Can you work these out from the model? Positions are in its coordinate system, mm. A direction names the side the tool comes from. Give positions to 0.01 mm unless a question says otherwise; leave off trailing zeros. Write each loop counter-clockwise with the first axis right and the second up, starting at its lowest first coordinate (ties: lowest second). Pieces come first, ordered by that corner, then holes.
1. Thinking about a two-plate mould opening in Y: for faces 1 (the flat face through (4, 0, 2)), 2 (the cylindrical face through (13.768, 5.555, 2.465)), 3 (the flat face through (4, 14, 0)), which applies, pulls with the +Y half, pulls with the -Y half, needs draft (parallel to the pull), parting line crosses it, or undercut?
2. On a 3-axis mill with a long thin cutter (end or side, diameter ignored), from which of +Z, -Z, +X, -X, +Y, -Y can I reach the whole of each face in a straight line? I mean faces 4 (the flat face through (28.266, 2, 2)), 5 (the flat face through (-22, 5, 2)), 6 (the flat face through (-24.734, 10, 2)), 7 (the flat face through (28.266, 18, 2)), 8 (the cylindrical face through (-15.303, 17.451, 2.465)). Say none if no direction works.
3. Suppose I cut it at C-C (z = 1.5). Please give me the cut outline in (x, y), and give its area (3 significant figures).
4. Suppose I cut it at B-B (x = -17.5). Please give me the cut outline in (y, z).
5. Suppose I cut it at A-A (y = 17). Please give me the cut outline in (x, z), and give its area (3 significant figures).
6. I'm going to push flat-ended pins straight in: pin 1 (1.5 mm diameter, centred on x = 30, z = 2, fed in from -Y); pin 2 (2.5 mm diameter, centred on x = 32, z = 2.5, fed in from +Y); pin 3 (1.5 mm diameter, centred on y = 17.5, z = 3.5, fed in from +X). Where does each tip first touch, or does it pass through?
7. Suppose I cut it at D-D (y = 20.5). Please give me the cut outline in (x, z).
8. If I drill on probe 1 along Y at (x, z) = (-17.5, 3.55); probe 2 along X at (y, z) = (16.25, 1.3); probe 3 along Y at (x, z) = (-16.5, 4.35), over which ranges is the centre line in solid material (lowest first)?
```python
from build123d import *

# Parameters (mm, degrees)
SKETCH1_R           = 1.5
SKETCH1_R_2         = 1.542918724
SKETCH1_R_3         = 1.500000001
BOSS_EXTRUDE1_DEPTH = 5
FILLET1_R           = 5
FILLET2_R           = 5


with BuildPart() as part:
    # Sketch1 → Boss-Extrude1 (new body)
    with BuildSketch(Plane.XY):
        Polygon((-19.733524355, 0), (28.266475645, 0), (28.266475645, 5), (33.266475645, 5), (33.266475645, 15), (28.266475645, 15), (28.266475645, 27), (-19.733524355, 27), (-19.733524355, 15), (-24.733524355, 15), (-24.733524355, 5), (-19.733524355, 5), align=None)
        with Locations((-16.733524355, 17)):
            Circle(SKETCH1_R, mode=Mode.SUBTRACT)
        with Locations((-16.733524356, 5.488599349)):
            Circle(SKETCH1_R_2, mode=Mode.SUBTRACT)
        with Locations((15.266475644, 17)):
            Circle(SKETCH1_R_3, mode=Mode.SUBTRACT)
        with Locations((15.266475644, 5.488599348)):
            Circle(SKETCH1_R_3, mode=Mode.SUBTRACT)
    extrude(amount=BOSS_EXTRUDE1_DEPTH)

    # Fillet1
    fillet1_edges = [part.edges().sort_by_distance(p)[0] for p in [
        (-19.733524355, 27, 2.5),
    ]]
    fillet(fillet1_edges, radius=FILLET1_R)

    # Fillet2
    fillet2_edges = [part.edges().sort_by_distance(p)[0] for p in [
        (28.266475645, 27, 2.5),
    ]]
    fillet(fillet2_edges, radius=FILLET2_R)


solid = part.part
```
Checks:
1. face 1: pulls with the -Y half
1. face 2: undercut
1. face 3: needs draft
2. face 4: +Z, -Z, +X, -Y
2. face 5: +Z, -Z, -X, -Y
2. face 6: +Z, -Z, -X, +Y, -Y
2. face 7: +Z, -Z, +X, +Y
2. face 8: +Z, -Z
3. outline: (-24.73, 5) - (-19.73, 5) - (-19.73, 0) - (28.27, 0) - (28.27, 5) - (33.27, 5) - (33.27, 15) - (28.27, 15) - (28.27, 22) arc R5 ccw to (23.27, 27) - (-14.73, 27) arc R5 ccw to (-19.73, 22) - (-19.73, 15) - (-24.73, 15) - close; hole circle Ø3.09 at (-16.73, 5.49); hole circle Ø3 at (-16.73, 17); hole circle Ø3 at (15.27, 5.49); hole circle Ø3 at (15.27, 17)
3. area: 1,360 mm2
4. outline: (0, 0) - (4.15, 0) - (4.15, 5) - (0, 5) - close; (6.83, 0) - (15.71, 0) - (15.71, 5) - (6.83, 5) - close; (18.29, 0) - (26.16, 0) - (26.16, 5) - (18.29, 5) - close
5. outline: (-19.73, 0) - (-18.23, 0) - (-18.23, 5) - (-19.73, 5) - close; (-15.23, 0) - (13.77, 0) - (13.77, 5) - (-15.23, 5) - close; (16.77, 0) - (28.27, 0) - (28.27, 5) - (16.77, 5) - close
5. area: 210 mm2
6. pin 1: stops at y = 5
6. pin 2: stops at y = 15
6. pin 3: stops at x = 28.27
7. outline: (-19.73, 0) - (28.27, 0) - (28.27, 5) - (-19.73, 5) - close
8. probe 1: y = 0 to 4.15, 6.83 to 15.71, 18.29 to 26.16
8. probe 2: x = -19.73 to -18.03, -15.43 to 13.97, 16.57 to 28.27
8. probe 3: y = 0 to 3.96, 7.01 to 15.52, 18.48 to 26.68
